from build123d import *

# Parameters (mm, degrees)
SKETCH2_W           = 21.7
SKETCH2_H           = 25.05
SKETCH2_RX          = 9.525
SKETCH2_RY          = 6.35
BOSS_EXTRUDE1_DEPTH = 12.7
SKETCH3_W           = 21.660653916
SKETCH3_H           = 25.05
BOSS_EXTRUDE2_DEPTH = 3
SKETCH5_W           = 18.892037138
SKETCH5_H           = 21.7
BOSS_EXTRUDE3_DEPTH = 2
SKETCH6_W           = 30
SKETCH6_H           = 21.7
BOSS_EXTRUDE4_DEPTH = 4
SKETCH7_W           = 21.7
SKETCH7_H           = 1
SKETCH7_W_2         = 3.175
SKETCH7_H_2         = 3
CUT_EXTRUDE2_DEPTH  = 23
SKETCH7_3_W         = 21.7
SKETCH7_3_H         = 7.272473706
CUT_EXTRUDE3_DEPTH  = 44.803879418
SKETCH11_R          = 1
CUT_EXTRUDE8_DEPTH  = 33.487034031
SKETCH15_W          = 3
SKETCH15_H          = 3
CUT_EXTRUDE9_DEPTH  = 28.443249292
CUT_EXTRUDE4_REACH  = 47.088
SKETCH9_R           = 1.5
SKETCH10_R          = 2
CUT_EXTRUDE7_DEPTH  = 1
FILLET5_R           = 6.35
FILLET6_R           = 2
FILLET7_R           = 2


with BuildPart() as part:
    # Sketch2 → Boss-Extrude1 (new body)
    with BuildSketch(Plane(origin=(16.497783942, 9.525, 0), x_dir=(0, 0, -1), z_dir=(0.8660254037844379, 0.5000000000000013, 0))):
        Rectangle(SKETCH2_W, SKETCH2_H)
        with Locations(Location((0, 0), (0, 0, 90))):
            Ellipse(SKETCH2_RX, SKETCH2_RY, mode=Mode.SUBTRACT)
    extrude(amount=-BOSS_EXTRUDE1_DEPTH)

    # Sketch3 → Boss-Extrude2 (add)
    with BuildSketch(Plane(origin=(5.499261314, 3.175, 0), x_dir=(0, 0, 1), z_dir=(-0.8660254037844379, -0.5000000000000014, 0))):
        with Locations((-0.019673042, 0)):
            Rectangle(SKETCH3_W, SKETCH3_H)
    extrude(amount=BOSS_EXTRUDE2_DEPTH)

    # Sketch5 → Boss-Extrude3 (add)
    with BuildSketch(Plane(origin=(0, 0, 0), x_dir=(-1, 0, 0), z_dir=(0, 1, 0))):
        with Locations((-13.314265373, 0)):
            Rectangle(SKETCH5_W, SKETCH5_H)
    extrude(amount=-BOSS_EXTRUDE3_DEPTH)

    # Sketch6 → Boss-Extrude4 (add)
    with BuildSketch(Plane.XZ.offset(2)):
        with Locations((18.868246804, 0)):
            Rectangle(SKETCH6_W, SKETCH6_H)
    extrude(amount=BOSS_EXTRUDE4_DEPTH)

    # Sketch7 → Cut-Extrude2 (cut)
    with BuildSketch(Plane(origin=(33.868246804, 0, 0), x_dir=(0, 0, -1), z_dir=(1, 0, 0))):
        with Locations((0, -2.5)):
            Rectangle(SKETCH7_W, SKETCH7_H)
        with Locations((0, -4.5)):
            Rectangle(SKETCH7_W_2, SKETCH7_H_2)
    extrude(amount=-CUT_EXTRUDE2_DEPTH, mode=Mode.SUBTRACT)

    # Sketch7<3> → Cut-Extrude3 (cut, through all)
    with BuildSketch(Plane(origin=(33.868246804, 0, 0), x_dir=(0, 0, -1), z_dir=(1, 0, 0))):
        with Locations((0, -9.636236853)):
            Rectangle(SKETCH7_3_W, SKETCH7_3_H)
    extrude(amount=-CUT_EXTRUDE3_DEPTH, mode=Mode.SUBTRACT)

    # Sketch11 → Cut-Extrude8 (cut, through all)
    with BuildSketch(Plane(origin=(19.672783942, 0.194872981, 0), x_dir=(0, 0, -1), z_dir=(-1, 0, 0))):
        with Locations(Location((0, -3.830865705, 0), (0, 0, 90))):
            Circle(SKETCH11_R)
    extrude(amount=CUT_EXTRUDE8_DEPTH, mode=Mode.SUBTRACT)

    # Sketch15 → Cut-Extrude9 (cut, symmetric)
    with BuildSketch(Plane(origin=(16.497783942, 9.525, 0), x_dir=(0.7757354378747654, -0.6310582623064579, 0), z_dir=(0.6310582623064579, 0.7757354378747654, 0))):
        with Locations((0, -8.35)):
            Rectangle(SKETCH15_W, SKETCH15_H)
    cut_extrude9 = extrude(amount=CUT_EXTRUDE9_DEPTH, both=True, mode=Mode.SUBTRACT)

    # Sketch9 → Cut-Extrude4 (cut, up to next)
    with BuildSketch(Plane(origin=(0, 0, -10.85), x_dir=(-1, 0, 0), z_dir=(0, 0, -1)), mode=Mode.PRIVATE) as cut_extrude4_sk1:
        with Locations((-14.332720433, 8.275)):
            Circle(SKETCH9_R)
    cut_extrude4_tool1 = extrude(cut_extrude4_sk1.sketch, amount=-CUT_EXTRUDE4_REACH, mode=Mode.PRIVATE) & part.part
    cut_extrude4 = cut_extrude4_tool1.solids().sort_by_distance((14.33272, 8.275, -10.85))[0]
    add(cut_extrude4, mode=Mode.SUBTRACT)

    # Sketch10 → Cut-Extrude7 (cut)
    with BuildSketch(Plane(origin=(0, 0, -10.85), x_dir=(-1, 0, 0), z_dir=(0, 0, -1))):
        with Locations((-14.332720433, 8.275)):
            Circle(SKETCH10_R)
    cut_extrude7 = extrude(amount=-CUT_EXTRUDE7_DEPTH, mode=Mode.SUBTRACT)

    # Mirror1: Cut-Extrude9, Cut-Extrude4, Cut-Extrude7 across plane
    add(cut_extrude9.mirror(Plane.XY), mode=Mode.SUBTRACT)
    add(cut_extrude4.mirror(Plane.XY), mode=Mode.SUBTRACT)
    add(cut_extrude7.mirror(Plane.XY), mode=Mode.SUBTRACT)

    # Fillet5
    fillet5_edges = [part.edges().sort_by_distance(p)[0] for p in [
        (33.868246804, -4.5, 10.85),
        (33.868246804, -4.5, -10.85),
        (22.760283942, -1, -10.85),
        (22.760283942, -1, 10.85),
        (4.736022628, 17.196968182, 10.85),
        (3.436984522, 16.446968182, -10.85),
    ]]
    fillet(fillet5_edges, radius=FILLET5_R)

    # Fillet6
    fillet6_edges = [part.edges().sort_by_distance(p)[0] for p in [
        (33.868246804, -4.5, 1.5875),
        (33.868246804, -4.5, -1.5875),
    ]]
    fillet(fillet6_edges, radius=FILLET6_R)

    # Fillet7
    # the kernel refuses this fillet: 2 mm, written as the material it takes off along each edge
    with BuildSketch(Plane(origin=(22.760283942, 0, 8.429393602), x_dir=(-1, 0, 0), z_dir=(0, 0, -1))) as fillet7_piece_1:
        with BuildLine():
            CenterArc((2, -1.571757441), FILLET7_R, 128.197977663, 51.802022337)
            Line((0, -1.571757441), (-0.04, -1.571757441))
            Line((-0.04, -1.571757441), (-0.04, 0))
            Line((-0.04, 0), (0, 0.04))
            ThreePointArc((0, 0.04), (0.381619343, 0.04), (0.73850346, 0.031435149))
            Line((0.73850346, 0.031435149), (0.763238686, 0))
        make_face()
    extrude(amount=16.858787203, mode=Mode.SUBTRACT)


solid = part.part
Geometry check sheet. Reference: the model listing, model coordinates, mm. A direction names the side the tool comes from. Round coordinates to 2 decimals unless told otherwise and drop trailing zeros. Write each loop counter-clockwise with the first axis right and the second up, starting at its lowest first coordinate (ties: lowest second). Pieces come first, ordered by that corner, then holes. Notation, with made-up numbers: (2, 36.5) - (24, 36.5) arc R28 ccw to (24, 74.5) - close; hole circle Ø4 at (22, 32). An arc over 180 degrees is marked (long way). One line per item, written item: value.
1. Cross-section at A-A on x = 25. Record the boundary of the cut face in (y, z).
The answers:
outline: (-6, -10.85) - (-3, -10.85) - (-3, -1.59) - (-6, -1.59) - close; (-6, 1.59) - (-3, 1.59) - (-3, 10.85) - (-6, 10.85) - close
2. Scan lines: L1, parallel to Z at x = 11, y = 8; L2, parallel to Z at x = 23, y = -4; L3, parallel to Y at x = 3.25, z = 0. Record each from-to range of solid material in increasing order.
The answers:
L1: z = -10.85 to -6.28, 6.28 to 10.85
L2: z = -10.85 to -1.59, 1.59 to 10.85
L3: y = 1.07 to 3.03, 5.03 to 7.07, 12.87 to 16.34
3. Depth check by flat-ended pin: pin 1 Ø6 at (x, z) = (7, -5) entering from +Y; pin 2 Ø2 at (y, z) = (5, -2) entering from +X; pin 3 Ø12 at (x, z) = (25.5, 5) entering from +Y (3 decimals). Enter the tip coordinate at first touch or a pass-through.
The answers:
pin 1: stops at y = 20.22
pin 2: stops at x = 5.02
pin 3: stops at y = 4.325
4. Mould release check, pull along Y, two halves, no side actions. Record for faces 1 (the face through (33.868, -4, 4)), 2 (the face through (10.868, -3, 0)), 3 (the face through (19, -6, 3)): released by +Y, released by -Y, zero draft, split by the parting line, or undercut.
The answers:
face 1: zero draft
face 2: undercut
face 3: released by -Y
5. Set-up check for faces 4 (the face through (23, -3, -6)), 5 (the face through (12.485, 7.509, 10.357)), 6 (the face through (19, 1.2, 10.3)), 7 (the face through (15.22, 10.33, 8.37)), 8 (the face through (10, 2, 6.85)): record each of +Z, -Z, +X, -X, +Y, -Y from which the full face is reachable in a straight line by a thin tool's end or side.
The answers:
face 4: +Z, -Z, +X
face 5: +Z
face 6: +Z, +X, +Y
face 7: +X
face 8: none
6. Cross-section at C-C on x = 31. Record the boundary of the cut face in (y, z).
The answers:
outline: (-6, -9.81) - (-3, -9.81) - (-3, -1.59) - (-6, -1.59) - close; (-6, 1.59) - (-3, 1.59) - (-3, 9.81) - (-6, 9.81) - close
7. Cross-section at B-B on z = 8.25. Record the boundary of the cut face in (x, y) (3 decimals), and give its area (3 significant figures).
The answers:
outline: (-2.749, 11.461) - (3.868, 0) - (3.868, -3.623) - (12.995, 7.596) arc R1.5 cw to (14.725, 9.723) - (15.695, 10.915) - (10.848, 19.311) - close; (5.802, -6) - (32.643, -6) - (32.643, -3) - (10.868, -3) - (10.868, -2) - (21.535, -2) - (21.535, 0.801) - (17.3, 8.135) - close
area: 348 mm^2
